Autodesk Inventor part; units mm, degrees
ref_plane "YZ Plane" through (0, 0, 0) normal (1, 0, 0) x (0, 1, 0)
ref_plane "XZ Plane" through (0, 0, 0) normal (0, 1, 0) x (-1, 0, 0)
ref_plane "XY Plane" through (0, 0, 0) normal (0, 0, 1) x (1, 0, 0)
sketch "Sketch1" plane through (0, 0, 0) normal (0, 0, 1) x (1, 0, 0)
  circle A0 centre (0, 0) radius 2.15
  line L0 (3.3137, 8) -> (8, 3.3137)
  line L1 (8, 3.3137) -> (8, -3.3137)
  line L2 (8, -3.3137) -> (3.3137, -8)
  line L3 (3.3137, -8) -> (-3.3137, -8)
  line L4 (-3.3137, -8) -> (-8, -3.3137)
  line L5 (-8, -3.3137) -> (-8, 3.3137)
  line L6 (-8, 3.3137) -> (-3.3137, 8)
  line L7 (-3.3137, 8) -> (3.3137, 8)
  dimension "d0" = 4.3
  dimension "d1" = 16
extrude "Extrusion1" add sketch "Sketch1" along normal blind 7
sketch "Sketch2" plane through (8, -3.3137, 0) normal (1, 0, 0) x (0, 0, -1)
  line L0 (0, 0) -> (-7, 0)
  line L1 (0, 6.6274) -> (0, 0)
  line L2 (0, 11.3137) -> (0, 6.6274)
  circle A0 centre (-16.7618, 16.384) radius 2.15
  circle A1 centre (-16.7618, 16.384) radius 4.15
  line L3 (0, 11.3137) -> (-7, 11.3137)
  line L4 (0, 11.3137) -> (-14.6531, 19.9583)
  line L5 (-7, 0) -> (-7, -4.6863)
  line L6 (-7, 0) -> (-19.7793, 13.5349)
  line L7 (-7, 1.1637) -> (-7, 5.4637)
  line L8 (-7, 3.3137) -> (-11, 3.3137)
  line L9 (-11, 3.3137) -> (-11, 7.0137)
  circle A2 centre (-16.7618, 16.384) radius 11
  point P0 (0, 3.3137)
  dimension "d4" = 4.3
  dimension "d6" = 2
  dimension "d17" = 4
  dimension "d18" = 3.7
  dimension "d19" = 22
extrude "Extrusion2" add sketch "Sketch2" against normal blind 4.8 contours L0 L6 L9 A2 L3 L2 L1 | L3 A2 L4 | L6 A2 L9 | A2 L6 A1 L4 | A1 picked at (-9.3805, 11.8131)
mirror "Mirror1" about plane through (0, 0, 0) normal (1, 0, 0) of "Extrusion2"
sketch "Sketch4" plane through (0, 0, 7) normal (0, 0, 1) x (1, 0, 0)
  circle A0 centre (0, 0) radius 3.7
  dimension "d14" = 7.4
extrude "Extrusion4" cut sketch "Sketch4" along normal through all
chamfer "Chamfer2" distance 1.6 angle 45 6 edges at (8, 15.6589, 20.0055) (8, 3.4538, 13.3896) (8, 12.3223, 7.3265) (-8, 3.4538, 13.3896) (-8, 15.6589, 20.0055) (-8, 12.3223, 7.3265)
chamfer "Chamfer3" distance 3.2 angle 45 1 edges at (0, 8, 7)
properties part number "kladka-midwheel-atTprofile"
The model under review builds one solid part; all positions refer to its coordinate system, in mm. A direction names the side the tool comes from. Give positions to 0.01 mm unless a question says otherwise; leave off trailing zeros. Write each loop counter-clockwise with the first axis right and the second up, starting at its lowest first coordinate (ties: lowest second). Pieces come first, ordered by that corner, then holes.
1. For P1, Ø3, axis at x = 1, y = -3.5, coming from the +Z side; P2, Ø4, axis at x = -1.5, y = -3, coming from the +Z side; P3, Ø3, axis at x = -1.5, z = 2, coming from the +Y side, all flat-tipped, find the tip position at first contact; note any pin that passes through.
2. Add section C-C, the plane y = 0. Write out the cut boundary in (x, z), plus the area to 3 significant figures.
3. Draft analysis for pull direction Y (two halves, no side actions). For faces 1 (the flat face through (3.2, -2.3, 7.4)), 2 (the cylindrical face through (5.634, 13.716, 14.711)), 3 (the flat face through (4.82, 12.26, 7.22)), state which applies: +Y half, -Y half, draft (parallel to the pull), parting line (faces both ways), or undercut.
4. Wall thickness on L1, parallel to X at y = 8.25, z = 9; L2, parallel to Y at x = 0, z = 2.25; L3, parallel to X at y = -1.25, z = 4: over which ranges is each line inside the solid? List them lowest first.
5. Add section A-A, the plane x = 0. Write out the cut boundary in (y, z).
6. Tool access review of faces 4 (the flat face through (3.2, 10, 13)), 5 (the cylindrical face through (-3.68, 0.4, 8.86)), 6 (the flat face through (-3.2, -2.4, 7.5)): name each direction out of +Z, -Z, +X, -X, +Y, -Y from which nothing blocks a thin tool from reaching the whole face with its end or side.
7. Add section D-D, the plane x = -4.5. Write out the cut boundary in (y, z), plus the area to 3 significant figures.
8. Add section B-B, the plane z = 7.75. Write out the cut boundary in (x, y), plus the area to 3 significant figures.
Worked answers:
1. P1: stops at z = 7
1. P2: stops at z = 8.29
1. P3: stops at y = 8
2. outline: (-8, 0) - (-2.15, 0) - (-2.15, 7) - (-3.7, 7) - (-3.7, 10.13) - (-6.4, 10.13) - (-8, 7.93) - close; (2.15, 0) - (8, 0) - (8, 7.93) - (6.4, 10.13) - (3.7, 10.13) - (3.7, 7) - (2.15, 7) - close
2. area: 105 mm2
3. face 1: draft
3. face 2: undercut
3. face 3: +Y half
4. L1: x = -8 to -3.2, 3.2 to 8
4. L2: y = -8 to -2.15, 2.15 to 8
4. L3: x = -8 to -1.75, 1.75 to 8
5. outline: (-8, 0) - (-2.15, 0) - (-2.15, 7) - (-8, 7) - close; (2.15, 0) - (8, 0) - (8, 3.8) - (4.8, 7) - (2.15, 7) - close
6. face 4: +Z, +Y
6. face 5: +Z
6. face 6: +Z, +Y, -Y
7. outline: (-6.81, 0) - (8, 0) - (16.64, 14.65) arc R4.15 ccw to (10.22, 19.78) - (-3.31, 7) - (-6.81, 7) - close; hole circle Ø4.3 at (13.07, 16.76)
7. area: 261 mm2
8. outline: (-8, -0.19) - (-6.4, -2.52) - (-3.2, -2.52) - (-3.2, -1.86) arc R3.7 cw to (-3.2, 1.86) - (-3.2, 12.57) - (-6.4, 12.57) - (-8, 10.71) - close; (3.2, -2.52) - (6.4, -2.52) - (8, -0.19) - (8, 10.71) - (6.4, 12.57) - (3.2, 12.57) - (3.2, 1.86) arc R3.7 cw to (3.2, -1.86) - close
8. area: 136 mm2
